Input: part model. Units: mm. Frame: model coordinates. A direction names the side the tool comes from. Coordinates: 2 decimals unless noted, no trailing zeros. Loops run counter-clockwise (first coordinate to the right, second up) from the corner with the lowest first, then second, coordinate; pieces in that order, holes last.
Item 1: Section C-C on y = 46. Return loops of the section in (x, z), and give its area (3 significant figures).
Item 2: Section B-B on z = -27. Return loops of the section in (x, y), and give its area (3 significant figures).
Item 3: Contact query for flat-ended pins moving along their axis: P1, Ø1.5, axis at x = 1.5, z = -61, coming from the +Y side; P2, Ø1.2, axis at x = 2, y = 22, coming from the -Z side; P3, Ø2, axis at x = 2.5, z = -5, coming from the -Y side; P4, Ø2, axis at x = 1.5, y = 18, coming from the +Z side. Output: stop coordinate, or through.
Item 4: Reachability of faces 4 (the flat face through (4, 70, -40)), 5 (the flat face through (2, 98, -66)) from +Z, -Z, +X, -X, +Y, -Y: full face, straight path, thin tool, end or side. Return the list, or none.
Item 5: Pull-direction query (Y, two-part tool) for faces 1 (the flat face through (2, 110, -65)), 2 (the flat face through (2, 138, -30)), 3 (the flat face through (0, 70, -40)); classes: released by +Y, released by -Y, zero draft, split by the parting line, or undercut.
Item 6: Section A-A on y = 15. Return loops of the section in (x, z), and give its area (3 significant figures).
Item 7: Ray query, line 1 along Y through (x, z) = (2.4, -30); line 2 along Z through (x, y) = (1.05, 64.5); line 3 along Y through (x, z) = (2.8, -4.5). Return the intervals inside material, ascending.
Item 8: Section D-D on x = 2.8. Give the number of separate pieces and of enclosed holes in the cut face, and give its area (3 significant figures).
```python
from build123d import *

# Parameters (mm, degrees)
SKETCH_1_W           = 60
SKETCH_1_H           = 50
SKETCH_1_R           = 2.1
EXTRUDE_1_DEPTH      = 4
EXTRUDE_2_DEPTH      = 4
EXTRUDE_4_DEPTH      = 4
SKETCH_10_W          = 9
SKETCH_10_H          = 10
SKETCH_10_W_2        = 3
EXTRUDE_5_DEPTH      = 4
CHAMFER_1_SIZE       = 10
SKETCH_11_R          = 25
SKETCH_11_R_2        = 2.1
CUT_EXTRUDE_7_DEPTH  = 10
CUT_EXTRUDE_8_DEPTH  = 10
EXTRUDE_6_DEPTH      = 4
SKETCH_16_R          = 1.6
CUT_EXTRUDE_9_DEPTH  = 4
CUT_EXTRUDE_11_DEPTH = 10
SKETCH_21_R          = 2.1
EXTRUDE_7_DEPTH      = 4
SKETCH_21_2_R        = 2.1
CUT_EXTRUDE_12_DEPTH = 10
CUT_EXTRUDE_13_DEPTH = 157.639713994
CUT_EXTRUDE_14_DEPTH = 157.639713994
SKETCH_24_R          = 1.5
CUT_EXTRUDE_15_DEPTH = 4
FILLET_1_R           = 1


with BuildPart() as part:
    # 草图1 → 凸台-拉伸1 (new body)
    with BuildSketch(Plane(origin=(0, 0, 0), x_dir=(0, 0, -1), z_dir=(1, 0, 0))):
        with Locations((30, 25)):
            Rectangle(SKETCH_1_W, SKETCH_1_H)
        with Locations((15, 4)):
            Circle(SKETCH_1_R, mode=Mode.SUBTRACT)
        with Locations((15, 46)):
            Circle(SKETCH_1_R, mode=Mode.SUBTRACT)
        with Locations(Location((45, 4, 0), (0, 0, 180))):
            Circle(SKETCH_1_R, mode=Mode.SUBTRACT)
        with Locations(Location((45, 46, 0), (0, 0, 180))):
            Circle(SKETCH_1_R, mode=Mode.SUBTRACT)
    extrude(amount=EXTRUDE_1_DEPTH)

    # 草图3 → 凸台-拉伸2 (add)
    with BuildSketch(Plane(origin=(4, 0, 0), x_dir=(0, 0, -1), z_dir=(1, 0, 0))):
        Polygon((0, 50), (-10, 38), (-10, 12), (0, 0), align=None)
        Polygon((70, 12), (60, 0), (60, 50), (70, 38), align=None)
    extrude(amount=-EXTRUDE_2_DEPTH)

    # 草图9 → 凸台-拉伸4 (add)
    with BuildSketch(Plane(origin=(4, 0, 0), x_dir=(0, 0, -1), z_dir=(1, 0, 0))):
        Polygon((60, 50), (65, 50), (65, 133), (60, 133), (0, 133), (-5, 133), (-5, 50), (0, 50), align=None)
        Polygon((-5, 50), (-5, 44), (0, 50), align=None)
        Polygon((65, 44), (60, 50), (65, 50), align=None)
    extrude(amount=-EXTRUDE_4_DEPTH)

    # 草图10 → 凸台-拉伸5 (add)
    with BuildSketch(Plane(origin=(4, 0, 0), x_dir=(0, 0, -1), z_dir=(1, 0, 0))):
        with Locations((-9.5, 128)):
            Rectangle(SKETCH_10_W, SKETCH_10_H)
        Polygon((-8, 123), (-14, 123), (-14, 88), (-8, 88), (-8, 98), align=None)
        with Locations((-6.5, 93)):
            Rectangle(SKETCH_10_W_2, SKETCH_10_H)
        with Locations((66.5, 93)):
            Rectangle(SKETCH_10_W_2, SKETCH_10_H)
        Polygon((68, 98), (68, 88), (74, 88), (74, 123), (68, 123), align=None)
        Polygon((65, 123), (68, 123), (74, 123), (74, 133), (65, 133), align=None)
    extrude(amount=-EXTRUDE_5_DEPTH)

    # 倒角1
    # the kernel refuses this chamfer: 10 mm, written as the material it takes off along each edge
    with BuildSketch(Plane(origin=(29.71682988, 88, -74), x_dir=(0, 0.9996219169112968, -0.027495876610586317), z_dir=(-1, 0, 0))) as chamfer_1_piece_1_section:
        Polygon((CHAMFER_1_SIZE * 0.999621916911, -CHAMFER_1_SIZE * 0.0274958766106), (-CHAMFER_1_SIZE * 0.0274958766106, -CHAMFER_1_SIZE * 0.999621916911), (0, 0), align=None)
    chamfer_1_piece_1 = extrude(amount=55.433659759, mode=Mode.PRIVATE)
    chamfer_1_piece_1 = split(chamfer_1_piece_1, bisect_by=Plane(origin=(2, 91.359007471, -65), z_dir=(0, 0, -1)), keep=Keep.TOP, mode=Mode.PRIVATE)
    add(chamfer_1_piece_1, mode=Mode.SUBTRACT)
    with BuildSketch(Plane(origin=(29.71682988, 88, 14), x_dir=(0, -0.027495876610586317, -0.9996219169112968), z_dir=(-1, 0, 0))) as chamfer_1_piece_2_section:
        Polygon((CHAMFER_1_SIZE * 0.999621916911, -CHAMFER_1_SIZE * 0.0274958766106), (-CHAMFER_1_SIZE * 0.0274958766106, -CHAMFER_1_SIZE * 0.999621916911), (0, 0), align=None)
    chamfer_1_piece_2 = extrude(amount=55.433659759, mode=Mode.PRIVATE)
    chamfer_1_piece_2 = split(chamfer_1_piece_2, bisect_by=Plane(origin=(2, 91.359007471, 5), z_dir=(0, 0, 1)), keep=Keep.TOP, mode=Mode.PRIVATE)
    add(chamfer_1_piece_2, mode=Mode.SUBTRACT)

    # 草图11 → 切除-拉伸7 (cut)
    with BuildSketch(Plane.ZY):
        with Locations((-30, 95)):
            Circle(SKETCH_11_R)
        with Locations((-9.493903346, 115.506096654)):
            Circle(SKETCH_11_R_2)
        with Locations((-22.494247692, 66.988151038)):
            Circle(SKETCH_11_R_2)
        with Locations((-58.011848962, 102.505752308)):
            Circle(SKETCH_11_R_2)
    extrude(amount=-CUT_EXTRUDE_7_DEPTH, mode=Mode.SUBTRACT)

    # 草图12 → 切除-拉伸8 (cut)
    with BuildSketch(Plane.ZY):
        with BuildLine():
            ThreePointArc((-32, 67.572823696), (-45.68490072, 72.411642614), (-55, 83.543560763))
            Line((-55, 83.543560763), (-55, 55))
            Line((-55, 55), (-32, 55))
            Line((-32, 55), (-32, 67.572823696))
        make_face()
        with BuildLine():
            ThreePointArc((-5, 83.543560763), (-9.75828346, 76.38487412), (-16.494247692, 71.044945114))
            Line((-16.494247692, 71.044945114), (-16.494247692, 55))
            Line((-16.494247692, 55), (-5, 55))
            Line((-5, 55), (-5, 83.543560763))
        make_face()
    extrude(amount=-CUT_EXTRUDE_8_DEPTH, mode=Mode.SUBTRACT)

    # 草图14 → 凸台-拉伸6 (add)
    with BuildSketch(Plane.ZY):
        with BuildLine():
            Line((-44.857355631, 55), (-39.575250068, 69.220849779))
            ThreePointArc((-39.575250068, 69.220849779), (-37.669905745, 68.591241115), (-35.723722086, 68.102249063))
            Line((-35.723722086, 68.102249063), (-40.590341434, 55))
            Line((-40.590341434, 55), (-44.857355631, 55))
        make_face()
    extrude(amount=-EXTRUDE_6_DEPTH)

    # 草图16 → 切除-拉伸9 (cut)
    with BuildSketch(Plane(origin=(4, 0, 0), x_dir=(0, 0, -1), z_dir=(1, 0, 0))):
        with Locations((-11, 128)):
            Circle(SKETCH_16_R)
        with Locations((-11, 108)):
            Circle(SKETCH_16_R)
        with Locations((71, 108)):
            Circle(SKETCH_16_R)
        with Locations((71, 128)):
            Circle(SKETCH_16_R)
    extrude(amount=-CUT_EXTRUDE_9_DEPTH, mode=Mode.SUBTRACT)

    # 草图20 → 切除-拉伸11 (cut)
    with BuildSketch(Plane.ZY):
        with BuildLine():
            ThreePointArc((8, 121), (9, 122), (8, 123))
            Line((8, 123), (8, 121))
        make_face()
        with BuildLine():
            Line((8, 100), (8, 98))
            ThreePointArc((8, 98), (9, 99), (8, 100))
        make_face()
        with BuildLine():
            Line((5, 121), (5, 123))
            ThreePointArc((5, 123), (4, 122), (5, 121))
        make_face()
        with BuildLine():
            ThreePointArc((5, 100), (4, 99), (5, 98))
            Line((5, 98), (5, 100))
        make_face()
        with BuildLine():
            Line((-65, 100), (-65, 98))
            ThreePointArc((-65, 98), (-64, 99), (-65, 100))
        make_face()
        with BuildLine():
            ThreePointArc((-65, 121), (-64, 122), (-65, 123))
            Line((-65, 123), (-65, 121))
        make_face()
        with BuildLine():
            ThreePointArc((-68, 100), (-69, 99), (-68, 98))
            Line((-68, 98), (-68, 100))
        make_face()
        with BuildLine():
            Line((-68, 121), (-68, 123))
            ThreePointArc((-68, 123), (-69, 122), (-68, 121))
        make_face()
    extrude(amount=-CUT_EXTRUDE_11_DEPTH, mode=Mode.SUBTRACT)

    # 草图21 → 凸台-拉伸7 (add)
    # profile 1 of 2: a face of its own
    with BuildSketch(Plane(origin=(4, 0, 0), x_dir=(0, 0, -1), z_dir=(1, 0, 0))):
        with BuildLine():
            Line((17.5, 138), (42.5, 138))
            ThreePointArc((42.5, 138), (46.035533906, 129.464466094), (37.5, 133))
            Line((37.5, 133), (22.5, 133))
            ThreePointArc((22.5, 133), (13.964466094, 129.464466094), (17.5, 138))
        make_face()
        with Locations((17.5, 133)):
            Circle(SKETCH_21_R, mode=Mode.SUBTRACT)
        with Locations((42.5, 133)):
            Circle(SKETCH_21_R, mode=Mode.SUBTRACT)
    # profile 2 of 2: a face of its own
    with BuildSketch(Plane(origin=(4, 0, 0), x_dir=(0, 0, -1), z_dir=(1, 0, 0))):
        with BuildLine():
            Line((42.5, 115), (17.5, 115))
            ThreePointArc((17.5, 115), (13.964466094, 123.535533906), (22.5, 120))
            Line((22.5, 120), (37.5, 120))
            ThreePointArc((37.5, 120), (46.035533906, 123.535533906), (42.5, 115))
        make_face()
        with Locations((17.5, 120)):
            Circle(SKETCH_21_R, mode=Mode.SUBTRACT)
        with Locations((42.5, 120)):
            Circle(SKETCH_21_R, mode=Mode.SUBTRACT)
    extrude(amount=-EXTRUDE_7_DEPTH)

    # 草图21<2> → 切除-拉伸12 (cut)
    with BuildSketch(Plane(origin=(4, 0, 0), x_dir=(0, 0, -1), z_dir=(1, 0, 0))):
        with Locations((17.5, 133)):
            Circle(SKETCH_21_2_R)
        with Locations((17.5, 120)):
            Circle(SKETCH_21_2_R)
        with Locations((42.5, 120)):
            Circle(SKETCH_21_2_R)
        with Locations((42.5, 133)):
            Circle(SKETCH_21_2_R)
    extrude(amount=-CUT_EXTRUDE_12_DEPTH, mode=Mode.SUBTRACT)

    # 草图22 → 切除-拉伸13 (cut, through all)
    with BuildSketch(Plane(origin=(4, 0, 0), x_dir=(0, 0, -1), z_dir=(1, 0, 0))):
        with BuildLine():
            Line((22.5, 133), (37.5, 133))
            ThreePointArc((37.5, 133), (38.316699867, 130.261387212), (40.5, 128.417424305))
            Line((40.5, 128.417424305), (40.5, 124.582575695))
            ThreePointArc((40.5, 124.582575695), (38.316699867, 122.738612788), (37.5, 120))
            Line((37.5, 120), (22.5, 120))
            ThreePointArc((22.5, 120), (21.683300133, 122.738612788), (19.5, 124.582575695))
            Line((19.5, 124.582575695), (19.5, 128.417424305))
            ThreePointArc((19.5, 128.417424305), (21.683300133, 130.261387212), (22.5, 133))
        make_face()
    extrude(amount=-CUT_EXTRUDE_13_DEPTH, mode=Mode.SUBTRACT)

    # 草图23 → 切除-拉伸14 (cut, through all)
    with BuildSketch(Plane(origin=(4, 0, 0), x_dir=(0, 0, -1), z_dir=(1, 0, 0))):
        with BuildLine():
            Line((0, 127), (8, 127))
            ThreePointArc((8, 127), (10, 125), (8, 123))
            Line((8, 123), (0, 123))
            ThreePointArc((0, 123), (-2, 125), (0, 127))
        make_face()
        with BuildLine():
            Line((60, 127), (52, 127))
            ThreePointArc((52, 127), (50, 125), (52, 123))
            Line((52, 123), (60, 123))
            ThreePointArc((60, 123), (62, 125), (60, 127))
        make_face()
    extrude(amount=-CUT_EXTRUDE_14_DEPTH, mode=Mode.SUBTRACT)

    # 草图24 → 切除-拉伸15 (cut)
    with BuildSketch(Plane.ZY):
        with Locations((-62, 35)):
            Circle(SKETCH_24_R)
        with Locations((-62, 15)):
            Circle(SKETCH_24_R)
        with Locations((2, 15)):
            Circle(SKETCH_24_R)
        with Locations((2, 35)):
            Circle(SKETCH_24_R)
        Polygon((-65, 44), (-65, 6), (-70, 12), (-70, 38), align=None)
        Polygon((5, 44), (5, 6), (10, 12), (10, 38), align=None)
        with BuildLine():
            Line((-48, 40), (-12, 40))
            ThreePointArc((-12, 40), (-10.585786438, 39.414213562), (-10, 38))
            Line((-10, 38), (-10, 12))
            ThreePointArc((-10, 12), (-10.585786438, 10.585786438), (-12, 10))
            Line((-12, 10), (-48, 10))
            ThreePointArc((-48, 10), (-49.414213562, 10.585786438), (-50, 12))
            Line((-50, 12), (-50, 38))
            ThreePointArc((-50, 38), (-49.414213562, 39.414213562), (-48, 40))
        make_face()
    extrude(amount=-CUT_EXTRUDE_15_DEPTH, mode=Mode.SUBTRACT)

    # 圆角1
    fillet_1_edges = [part.edges().sort_by_distance(p)[0] for p in [
        (2, 133, -74),
        (2, 98, -74),
        (2, 89, -65),
        (2, 83.543560763, -55),
        (2, 67.572823696, -32),
        (2, 55, -32),
        (2, 55, -55),
        (2, 71.044945114, -16.494247692),
        (2, 83.543560763, -5),
        (2, 55, -5),
        (2, 55, -16.494247692),
        (2, 69.220849779, -39.575250068),
        (2, 68.102249063, -35.723722086),
        (2, 55, -40.590341434),
        (2, 55, -44.857355631),
        (2, 115.397795547, -15.545591094),
        (2, 115.397795547, -44.454408906),
        (2, 133, 14),
    ]]
    fillet(fillet_1_edges, radius=FILLET_1_R)


solid = part.part
```
Results found:
1. outline: (0, -65) - (4, -65) - (4, -47.1) - (0, -47.1) - close; (0, -42.9) - (4, -42.9) - (4, -17.1) - (0, -17.1) - close; (0, -12.9) - (4, -12.9) - (4, 5) - (0, 5) - close
1. area: 246 mm2
2. outline: (0, 0) - (4, 0) - (4, 10) - (0, 10) - close; (0, 40) - (4, 40) - (4, 70.18) - (0, 70.18) - close; (0, 115) - (4, 115) - (4, 120) - (0, 120) - close; (0, 133) - (4, 133) - (4, 138) - (0, 138) - close
2. area: 201 mm2
3. P1: stops at y = 133
3. P2: stops at z = -65
3. P3: stops at y = 0
3. P4: stops at z = 5
4. face 4: +Z, -Z, +X, +Y, -Y
4. face 5: +X, -X
5. face 1: undercut
5. face 2: released by +Y
5. face 3: zero draft
6. outline: (0, -65) - (4, -65) - (4, -63.5) - (0, -63.5) - close; (0, -60.5) - (4, -60.5) - (4, -50) - (0, -50) - close; (0, -10) - (4, -10) - (4, 0.5) - (0, 0.5) - close; (0, 3.5) - (4, 3.5) - (4, 5) - (0, 5) - close
6. area: 96.0 mm2
7. line 1: y = 0 to 10, 40 to 70, 115 to 120, 133 to 138
7. line 2: z = -65 to -55, -41.33 to -37.06, -32 to -16.49, -5 to 5
7. line 3: y = 0 to 123, 127 to 133
8. separate pieces: 1
8. enclosed holes: 29
8. area: 5,820 mm2
